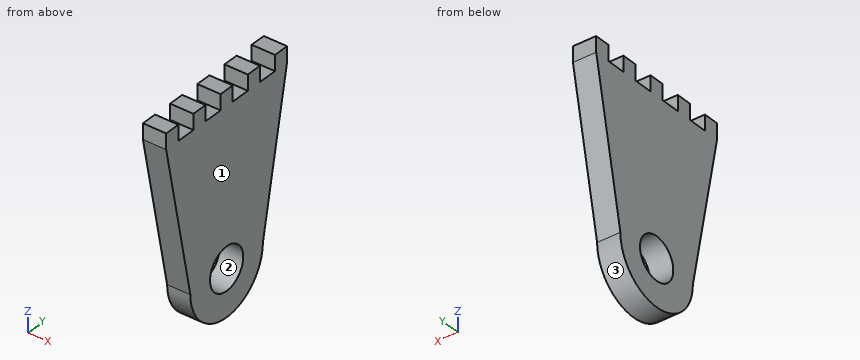
```python
from build123d import *

# Parameters (mm, degrees)
SKETCH1_R           = 2.75
BOSS_EXTRUDE1_DEPTH = 3


with BuildPart() as part:
    # Sketch1 → Boss-Extrude1 (new body)
    with BuildSketch(Plane(origin=(0, 0, 0), x_dir=(0, 0, -1), z_dir=(1, 0, 0))):
        with BuildLine():
            Line((-20, 5.5), (-22, 5.5))
            Line((-22, 5.5), (-22, 3.5))
            Line((-22, 3.5), (-20, 3.5))
            Line((-20, 3.5), (-20, 1))
            Line((-20, 1), (-22, 1))
            Line((-22, 1), (-22, -1))
            Line((-22, -1), (-20, -1))
            Line((-20, -1), (-20, -3.5))
            Line((-20, -3.5), (-22, -3.5))
            Line((-22, -3.5), (-22, -5.5))
            Line((-22, -5.5), (-20, -5.5))
            Line((-20, -5.5), (-20, -8))
            Line((-20, -8), (-22, -8))
            Line((-22, -8), (-22, -10))
            Line((-22, -10), (-20, -10))
            Line((-20, -10), (0, -6))
            ThreePointArc((0, -6), (6, 0), (0, 6))
            Line((0, 6), (-20, 10))
            Line((-20, 10), (-22, 10))
            Line((-22, 10), (-22, 8))
            Line((-22, 8), (-20, 8))
            Line((-20, 8), (-20, 5.5))
        make_face()
        Circle(SKETCH1_R, mode=Mode.SUBTRACT)
    extrude(amount=BOSS_EXTRUDE1_DEPTH)


solid = part.part
```
CAD build for the part. Positions are in the model's coordinates, mm. Face numbers are marked on the shaded views. Give positions to 0.01 mm unless a question says otherwise; leave off trailing zeros. Order: outer loops, then holes, each group sorted by start corner. A loop starts at its lowest first (then second) coordinate and runs counter-clockwise, first axis right, second up. Notation, with made-up numbers: M -10,37 L 24,37 A22 cw 24,74 Z; hole C 81,1.25 d8. An arc over 180 degrees is marked long. Put each result on its own line as item: value. Start each with the question number.
(1) Saw through at A-A, the plane y = 0. Write the cut outline in (x, z), then the cut area to 3 significant figures.
(2) Drill centre lines: line 1 along Y through (x, z) = (0.9, 0.5); line 2 along Y through (x, z) = (0.4, -1.25); line 3 along Z through (x, y) = (0.2, 0.5). Where is each one in solid material? Low to high.
(3) Saw through at B-B, the plane x = 1.25. Write the cut outline in (y, z).
(4) Saw through at C-C, the plane z = -1. Write the cut outline in (x, y).
(5) Flat gauge pins, fed straight in: pin 1 Ø1.2 at (x, y) = (1, 7) entering from +Z; pin 2 Ø1.5 at (x, z) = (2, 0.5) entering from -Y; pin 3 Ø6 at (y, z) = (-1, 0.5) entering from -X. Where does each tip first touch, or does it go through?
(6) Saw through at D-D, the plane z = 7.5. Write the cut outline in (x, y).
(7) Mould opens along Z. For the marked faces 1, 2 and 3 say: +Z half, -Z half, draft (parallel to the pull), parting line (faces both ways), or undercut.
Check result:
1. outline: M 0,-6 L 3,-6 L 3,-2.75 L 0,-2.75 Z; M 0,2.75 L 3,2.75 L 3,22 L 0,22 Z
1. area: 67.5 mm2
2. line 1: y = -6.1 to -2.7, 2.7 to 6.1
2. line 2: y = -5.87 to -2.45, 2.45 to 5.87
2. line 3: z = -5.98 to -2.7, 2.7 to 22
3. outline: M -10,20 L -6,0 A6 ccw 6,0 L 10,20 L 10,22 L 8,22 L 8,20 L 5.5,20 L 5.5,22 L 3.5,22 L 3.5,20 L 1,20 L 1,22 L -1,22 L -1,20 L -3.5,20 L -3.5,22 L -5.5,22 L -5.5,20 L -8,20 L -8,22 L -10,22 Z; hole C 0,0 d5.5
4. outline: M 0,-5.92 L 3,-5.92 L 3,-2.56 L 0,-2.56 Z; M 0,2.56 L 3,2.56 L 3,5.92 L 0,5.92 Z
5. pin 1: stops at z = 20
5. pin 2: stops at y = -6.25
5. pin 3: stops at x = 0
6. outline: M 0,-7.5 L 3,-7.5 L 3,7.5 L 0,7.5 Z
7. face 1: draft
7. face 2: undercut
7. face 3: -Z half
